Autodesk Inventor part; units mm, degrees
ref_plane "YZ Plane" through (0, 0, 0) normal (1, 0, 0) x (0, 1, 0)
ref_plane "XZ Plane" through (0, 0, 0) normal (0, 1, 0) x (-1, 0, 0)
ref_plane "XY Plane" through (0, 0, 0) normal (0, 0, 1) x (1, 0, 0)
sketch "スケッチ1" plane through (0, 0, 0) normal (0, 0, 1) x (1, 0, 0)
  circle A0 centre (-55, 0) radius 8.025 construction
  circle A1 centre (0, 0) radius 1.25 construction
  arc A2 (-44.5788, 6) -> (-63.6661, 8.3366) centre (-55, 0) ccw construction
  line L0 (-63.6661, 8.3366) -> (-109.1623, -38.9576) construction
  line L1 (-102.7709, -46.5745) -> (-48.2949, -9.9821) construction
  arc A3 (-48.2949, -9.9821) -> (-44.5788, -6) centre (-55, 0) ccw construction
  line L2 (-44.5788, -6) -> (-5.2915, -6) construction
  arc A4 (-5.2915, -6) -> (-5.2915, 6) centre (0, 0) ccw construction
  line L3 (-5.2915, 6) -> (-44.5788, 6) construction
  circle A5 centre (0, 0) radius 1.25
  circle A6 centre (-30, 0) radius 1.25
  circle A7 centre (-12, 0) radius 1.25
  circle A8 centre (-21, 0) radius 1.25
  line L4 (-30, 0) -> (0, 0)
  line L5 (-30, 0) -> (-50, 0)
  line L6 (-50, 0) -> (-30, 0)
  circle A9 centre (-50, 0) radius 1.25
  circle A10 centre (-50, 0) radius 4.025 construction
  circle A11 centre (-50, 0) radius 7.125 construction
  circle A12 centre (-57.7782, -7.7782) radius 1.25
  circle A13 centre (-57.7782, -7.7782) radius 3 construction
  line L7 (-50, 0) -> (-57.7782, -7.7782) construction
  line L8 (-53.1753, 3.2604) -> (-60.169, -5.9659)
  line L9 (-55.3874, -9.5904) -> (-46.209, 2.5181)
  arc A14 (-46.209, 2.5181) -> (-53.1753, 3.2604) centre (-50, 0) ccw
  arc A15 (-60.169, -5.9659) -> (-55.3874, -9.5904) centre (-57.7782, -7.7782) ccw
  line L10 (-50, 0) -> (0, 0) construction
  line L11 (-50, -4.5) -> (0, -4.5)
  line L12 (0, 4.5) -> (-50, 4.5)
  arc A16 (-50, 4.5) -> (-50, -4.5) centre (-50, 0) ccw
  arc A17 (0, -4.5) -> (0, 4.5) centre (0, 0) ccw
  line L13 (-57.7782, -10.7782) -> (-54.9706, -10.7782)
  line L14 (-54.9706, -10.7782) -> (-48.1997, -4.5)
  line L15 (-50, 0) -> (-57.7782, -7.7782)
  circle A18 centre (-12, 0) radius 4.5
  point P0 (-53.8891, -3.8891)
  point P1 (-25, 0)
  point P2 (-48.7574, -3)
  point P3 (-49.3198, 4.5)
  point P4 (-53.5862, 2.7184)
  point P5 (-51.3675, -4.2872)
  point P6 (-12, -4.5)
  point P7 (-12, 4.5)
  dimension "d0" = 20
  dimension "d2" = 2.5
  dimension "d3" = 8.05
  dimension "d4" = 3.1
  dimension "d5" = 30
  dimension "d6" = 2.5
  dimension "d7" = 2.5
  dimension "d8" = 2.5
  dimension "d9" = 2.5
  dimension "d11" = 9
  dimension "d13" = 2.5
  dimension "d14" = 6
  dimension "d15" = 6
  dimension "d16" = 9
  dimension "d21" = 135
  dimension "d22" = 10
  dimension "d30" = 9
  dimension "d31" = 11
extrude "押し出し1" add sketch "スケッチ1" along normal blind 3 contours L4 A8 A18 L11 A16 L9 L5 A6 | A6 L5 L9 A14 L12 A18 L4 A8 | L9 A16 L15 A9 L5 | L5 A9 L15 A16 L12 A14 L9 | A16 L11 L14 L13 A15 L9 | L9 A15 L8 A16 | A18 L4 A7 | L4 A7 A18 | L12 A16 L8 A14
fillet "フィレット1" radius 1.05 1 edges at (-48.1997, -4.5, 1.5)
sketch "スケッチ2" plane through (0, 0, 3) normal (0, 0, 1) x (1, 0, 0)
  arc A0 (-60.7927, -6.5251) -> (-59.7797, -5.8711) centre (-60.7525, -5.4759) ccw
  arc A1 (-55.3849, -4.4725) -> (-59.7797, -5.8711) centre (-57.0004, -7.0004) ccw
  arc A2 (-55.3849, -4.4725) -> (-43.7567, 3.1657) centre (-50, 0) ccw
  arc A3 (-44.0452, 4.6286) -> (-43.7567, 3.1657) centre (-43.1001, 4.055) ccw
  line L0 (-44.0452, 4.6286) -> (-41.5381, 8.9709)
  arc A4 (-41.5381, 8.9709) -> (-46.5567, 11.6351) centre (-44, 10.3923) ccw
  line L1 (-46.5567, 11.6351) -> (-49.0637, 7.2927)
  arc A5 (-50.5985, 6.9744) -> (-49.0637, 7.2927) centre (-49.9731, 7.8177) ccw
  arc A6 (-50.5985, 6.9744) -> (-50.2678, 6.9949) centre (-50, 0) ccw
  circle A7 centre (-50, 0) radius 4.025
  circle A8 centre (-50, 0) radius 1.25
  circle A9 centre (-39, 0) radius 4
  line L2 (-50, 0) -> (-38.3804, 0)
  circle A10 centre (-39, 0) radius 1.25
  circle A11 centre (-30, 0) radius 1.25
  point P0 (0, 0)
  point P1 (-43.3711, 2.3255)
  point P2 (-43, 0)
  point P3 (-49.3534, 6.9701)
  point P4 (-44.1966, 3.9141)
  point P5 (-43.7567, 3.1657)
  dimension "d23" = 12
  dimension "d24" = 8
  dimension "d27" = 2.5
  dimension "d28" = 9
  dimension "d29" = 7
extrude "押し出し2" cut sketch "スケッチ2" against normal blind 3 contours A10
thread "ねじ1"
thread "ねじ2"
thread "ねじ3"
thread "ねじ4"
thread "ねじ5"
thread "ねじ6"
properties part number "中間節アーム先端締結パーツ外" material "アルミニウム 7075"
Can you work these out from the model? Positions are in its coordinate system, mm. A direction names the side the tool comes from. Coordinates: 2 decimals unless noted, no trailing zeros. Loops run counter-clockwise (first coordinate to the right, second up) from the corner with the lowest first, then second, coordinate; pieces in that order, holes last. Notation, with made-up numbers: M 54,54.5 L 84,54.5 A26 ccw 84,92.5 Z; hole C 19,-28 d9. An arc over 180 degrees is marked long. Put each result on its own line as item: value. Start each with the question number.
(1) Will these pins go through, and if not, where does the flat tip stop? pin 1 Ø0.9 at (x, z) = (-21.5, 1) entering from +Y; pin 2 Ø1.5 at (x, y) = (-39, 0) entering from +Z; pin 3 Ø1 at (x, z) = (-27.5, 2.5) entering from -Y; pin 4 Ø1 at (y, z) = (-7, 1) entering from -X.
(2) Imagine slicing it at A-A on x = -30. List the corners of the cut face in (y, z) for me, and give its area (3 significant figures).
(3) Imagine slicing it at B-B on y = 0. List the corners of the cut face in (x, z) for me, and give its area (3 significant figures).
(4) Imagine slicing it at D-D on x = -50. List the corners of the cut face in (y, z) for me.
(5) Imagine slicing it at C-C on z = 1.1. List the corners of the cut face in (x, y) for me.
(6) Which directions (+Z, -Z, +X, -X, +Y, -Y) give clear straight access to the entire face, cutting with the end or side of a thin tool? Please do faces 5 (the face through (-30, 4.5, 1)), 6 (the face through (-56.623, -1.288, 1.479)).
(7) We'd pull the mould along Y, two halves only. Please class faces 1 (the face through (-19.845, 0.479, 1.479)), 2 (the face through (-30, -4.5, 1)), 3 (the face through (-60.444, -9.155, 1.479)), 4 (the face through (-13.25, -0.05, 1.48)): +Y half, -Y half, draft (parallel to the pull), parting line (faces both ways), or undercut.
(8) I need wall thicknesses on probe 1 along Y at (x, z) = (-21, 0.75); probe 2 along Y at (x, z) = (-22.5, 0.3); probe 3 along Y at (x, z) = (-49.5, 1.85). Which ranges of each line are inside material? Lowest first, please.
Worked answers:
1. pin 1: stops at y = 4.5
1. pin 2: passes through
1. pin 3: stops at y = -4.5
1. pin 4: stops at x = -60.77
2. outline: M -4.5,0 L -1.25,0 L -1.25,3 L -4.5,3 Z; M 1.25,0 L 4.5,0 L 4.5,3 L 1.25,3 Z
2. area: 19.5 mm2
3. outline: M -55.65,0 L -51.25,0 L -51.25,3 L -55.65,3 Z; M -48.75,0 L -40.25,0 L -40.25,3 L -48.75,3 Z; M -37.75,0 L -31.25,0 L -31.25,3 L -37.75,3 Z; M -28.75,0 L -22.25,0 L -22.25,3 L -28.75,3 Z; M -19.75,0 L -13.25,0 L -13.25,3 L -19.75,3 Z; M -10.75,0 L -7.5,0 L -7.5,3 L -10.75,3 Z
3. area: 107 mm2
4. outline: M -6.17,0 L -1.25,0 L -1.25,3 L -6.17,3 Z; M 1.25,0 L 4.55,0 L 4.55,3 L 1.25,3 Z
5. outline: M -60.17,-5.97 A3 ccw -57.78,-10.78 L -54.97,-10.78 L -48.5,-4.78 A1.05 cw -47.79,-4.5 L -12,-4.5 A4.5 ccw -12,4.5 L -49.32,4.5 A4.55 ccw -53.18,3.26 Z; hole C -57.78,-7.78 d2.5; hole C -50,0 d2.5; hole C -39,0 d2.5; hole C -30,0 d2.5; hole C -21,0 d2.5; hole C -12,0 d2.5
6. face 5: +Z, -Z, +X, +Y
6. face 6: +Z, -Z, -X, +Y
7. face 1: undercut
7. face 2: -Y half
7. face 3: parting line
7. face 4: undercut
8. probe 1: y = -4.5 to -1.25, 1.25 to 4.5
8. probe 2: y = -4.5 to 4.5
8. probe 3: y = -5.71 to -1.15, 1.15 to 4.52
